Model file for the job. Use its own axes, mm. A direction names the side the tool comes from. Give positions to 0.01 mm unless a question says otherwise; leave off trailing zeros. Write each loop counter-clockwise with the first axis right and the second up, starting at its lowest first coordinate (ties: lowest second). Pieces come first, ordered by that corner, then holes.
```python
from build123d import *

# Parameters (mm, degrees)
SKETCH1_W           = 3.5
SKETCH1_H           = 1
SKETCH1_W_2         = 4
BOSS_EXTRUDE1_DEPTH = 1.3
SKETCH1_7_W         = 3.5
SKETCH1_7_H         = 1
BOSS_EXTRUDE3_DEPTH = 1
SKETCH1_8_W         = 4
SKETCH1_8_H         = 1
BOSS_EXTRUDE4_DEPTH = 1
FILLET2_R           = 1
SKETCH5_W           = 1.00602476
SKETCH5_H           = 0.93
BOSS_EXTRUDE5_DEPTH = 4
SKETCH7_W           = 1.00602476
SKETCH7_H           = 0.93
BOSS_EXTRUDE6_DEPTH = 3.5
BOSS_EXTRUDE7_DEPTH = 1
BOSS_EXTRUDE8_START = 1.3
BOSS_EXTRUDE8_DEPTH = 0.7
FILLET6_START       = -4.975
FILLET6_DEPTH       = 9.95
FILLET7_R           = 0.15
SKETCH10_W          = 0.9
SKETCH10_H          = 0.9
BOSS_EXTRUDE9_DEPTH = 4
CHAMFER2_SIZE       = 0.8
CHAMFER2_SIZE2      = 0.373046127
FILLET9_R           = 0.15
FILLET10_R          = 0.1
CHAMFER5_SIZE       = 1


with BuildPart() as part:
    # Sketch1 → Boss-Extrude1 (new body)
    # profile 1 of 4: a face of its own
    with BuildSketch(Plane(origin=(0, 0, 0), x_dir=(1, 0, 0), z_dir=(0, 1, 0))):
        with BuildLine():
            Line((0, 9.25), (-4.925, 9.25))
            Line((-4.925, 9.25), (-4.925, 8.25))
            Line((-4.925, 8.25), (-8.425, 8.25))
            Line((-8.425, 8.25), (-8.425, 9.25))
            Line((-8.425, 9.25), (-15.925, 9.25))
            ThreePointArc((-15.925, 9.25), (-18.399873734, 8.224873734), (-19.425, 5.75))
            Line((-19.425, 5.75), (-19.425, -8.25))
            ThreePointArc((-19.425, -8.25), (-19.132106781, -8.957106781), (-18.425, -9.25))
            Line((-18.425, -9.25), (-8, -9.25))
            Line((-8, -9.25), (-4.975, -9.25))
            Line((-4.975, -9.25), (-4.975, -9.15))
            Line((-4.975, -9.15), (-2, -9.15))
            Line((-2, -9.15), (-2, -8.75))
            Line((-2, -8.75), (-2, -8.25))
            Line((-2, -8.25), (-7.5, -8.25))
            ThreePointArc((-7.5, -8.25), (-8, -7.75), (-7.5, -7.25))
            Line((-7.5, -7.25), (7.5, -7.25))
            ThreePointArc((7.5, -7.25), (8, -7.75), (7.5, -8.25))
            Line((7.5, -8.25), (2, -8.25))
            Line((2, -8.25), (2, -8.75))
            Line((2, -8.75), (2, -9.15))
            Line((2, -9.15), (4.975, -9.15))
            Line((4.975, -9.15), (4.975, -9.25))
            Line((4.975, -9.25), (8, -9.25))
            Line((8, -9.25), (18.425, -9.25))
            ThreePointArc((18.425, -9.25), (19.132106781, -8.957106781), (19.425, -8.25))
            Line((19.425, -8.25), (19.425, 5.75))
            ThreePointArc((19.425, 5.75), (18.399873734, 8.224873734), (15.925, 9.25))
            Line((15.925, 9.25), (9.675, 9.25))
            Line((9.675, 9.25), (9.675, 8.25))
            Line((9.675, 8.25), (5.675, 8.25))
            Line((5.675, 8.25), (5.675, 9.25))
            Line((5.675, 9.25), (0, 9.25))
        make_face()
        with BuildLine():
            Line((-13.05, -6.65), (-14.5, -6.65))
            ThreePointArc((-14.5, -6.65), (-16.214733944, -5.939733944), (-16.925, -4.225))
            ThreePointArc((-16.925, -4.225), (-16.214733944, -2.510266056), (-14.5, -1.8))
            Line((-14.5, -1.8), (-13.05, -1.8))
            ThreePointArc((-13.05, -1.8), (-11.335266056, -2.510266056), (-10.625, -4.225))
            ThreePointArc((-10.625, -4.225), (-11.335266056, -5.939733944), (-13.05, -6.65))
        make_face(mode=Mode.SUBTRACT)
        with BuildLine():
            ThreePointArc((-16.925, 4.225), (-16.214733944, 5.939733944), (-14.5, 6.65))
            Line((-14.5, 6.65), (-13.05, 6.65))
            ThreePointArc((-13.05, 6.65), (-11.335266056, 5.939733944), (-10.625, 4.225))
            ThreePointArc((-10.625, 4.225), (-11.335266056, 2.510266056), (-13.05, 1.8))
            Line((-13.05, 1.8), (-14.5, 1.8))
            ThreePointArc((-14.5, 1.8), (-16.214733944, 2.510266056), (-16.925, 4.225))
        make_face(mode=Mode.SUBTRACT)
    # profile 2 of 4: a face of its own
    with BuildSketch(Plane(origin=(0, 0, 0), x_dir=(1, 0, 0), z_dir=(0, 1, 0))):
        with Locations((-6.675, 8.75)):
            Rectangle(SKETCH1_W, SKETCH1_H)
    # profile 3 of 4: a face of its own
    with BuildSketch(Plane(origin=(0, 0, 0), x_dir=(1, 0, 0), z_dir=(0, 1, 0))):
        with Locations((7.675, 8.75)):
            Rectangle(SKETCH1_W_2, SKETCH1_H)
    # profile 4 of 4: a face of its own
    with BuildSketch(Plane(origin=(0, 0, 0), x_dir=(1, 0, 0), z_dir=(0, 1, 0))):
        Polygon((-2, -8.75), (-2, -9.15), (2, -9.15), (2, -8.75), (2, -8.25), (-2, -8.25), align=None)
    extrude(amount=BOSS_EXTRUDE1_DEPTH)

    # Sketch1<7> → Boss-Extrude3 (add)
    with BuildSketch(Plane(origin=(0, 0, 0), x_dir=(1, 0, 0), z_dir=(0, 1, 0))):
        with Locations((-6.675, 8.75)):
            Rectangle(SKETCH1_7_W, SKETCH1_7_H)
    extrude(amount=-BOSS_EXTRUDE3_DEPTH)

    # Sketch1<8> → Boss-Extrude4 (add)
    with BuildSketch(Plane(origin=(0, 0, 0), x_dir=(1, 0, 0), z_dir=(0, 1, 0))):
        with Locations((7.675, 8.75)):
            Rectangle(SKETCH1_8_W, SKETCH1_8_H)
    extrude(amount=-BOSS_EXTRUDE4_DEPTH)

    # Fillet2
    fillet2_edges = [part.edges().sort_by_distance(p)[0] for p in [
        (7.675, -1, -8.25),
        (-6.675, -1, -8.25),
    ]]
    fillet(fillet2_edges, radius=FILLET2_R - 0.0001)  # a hair under: the kernel refuses the full size

    # Sketch5 → Boss-Extrude5 (add)
    with BuildSketch(Plane.ZY.offset(-9.675)):
        with Locations((-9.75301238, -0.535)):
            Rectangle(SKETCH5_W, SKETCH5_H)
    extrude(amount=BOSS_EXTRUDE5_DEPTH)

    # Sketch7 → Boss-Extrude6 (add)
    with BuildSketch(Plane.ZY.offset(8.425)):
        with Locations((-9.75301238, -0.535)):
            Rectangle(SKETCH7_W, SKETCH7_H)
    extrude(amount=-BOSS_EXTRUDE6_DEPTH)

    # Sketch1<12> → Boss-Extrude7 (add)
    with BuildSketch(Plane(origin=(0, 0, 0), x_dir=(1, 0, 0), z_dir=(0, 1, 0))):
        Polygon((-2, -8.75), (-2, -9.15), (2, -9.15), (2, -8.75), (2, -8.25), (-2, -8.25), align=None)
    extrude(amount=-BOSS_EXTRUDE7_DEPTH)

    # Sketch1<13> → Boss-Extrude8 (add)
    with BuildSketch(Plane(origin=(0, 0, 0), x_dir=(1, 0, 0), z_dir=(0, 1, 0)).offset(BOSS_EXTRUDE8_START)):
        Polygon((-4.975, -9.15), (-4.975, -9.25), (0, -9.25), (4.975, -9.25), (4.975, -9.15), (2, -9.15), (-2, -9.15), align=None)
    extrude(amount=-BOSS_EXTRUDE8_DEPTH)

    # Fillet6: read off the stored shape, not the designer's step
    # Fillet6 outline → Fillet6 (add)
    with BuildSketch(Plane.YZ.offset(FILLET6_START)):
        with BuildLine():
            Line((0.6, 9.15), (0.6, 9.25))
            add(Edge.make_bspline(
                [(0.6, 9.25), (0.59163758, 9.15), (0.002086963, 9.15)],
                knots=[0, 0, 0, 1, 1, 1], degree=2, weights=[1, 0.735980072, 1]))
            Line((0.002086963, 9.15), (0.6, 9.15))
        make_face()
    extrude(amount=FILLET6_DEPTH)

    # Fillet7
    # the kernel refuses this fillet: 0.15 mm, written as the material it adds along each edge
    with BuildSketch(Plane(origin=(-4.975, 0, 9.15), x_dir=(1, 0, 0), z_dir=(0, 1, 0))) as fillet7_piece_1:
        with BuildLine():
            CenterArc((0.141421356, -0.15), FILLET7_R, 90, 70.528779366)
            Line((0, -0.1), (-0.002828427, -0.099))
            ThreePointArc((-0.002828427, -0.099), (-0.003, -0.05), (-0.003, 0))
            Line((-0.003, 0), (0, 0.003))
            Line((0, 0.003), (0.141421356, 0.003))
            Line((0.141421356, 0.003), (0.141421356, 0))
        make_face()
    extrude(amount=0.603127727)
    with BuildSketch(Plane(origin=(4.975, 0, 9.15), x_dir=(0, 0, 1), z_dir=(0, 1, 0))) as fillet7_piece_2:
        with BuildLine():
            CenterArc((0.15, -0.141421356), FILLET7_R, 109.471220634, 70.528779366)
            Line((0, -0.141421356), (-0.003, -0.141421356))
            Line((-0.003, -0.141421356), (-0.003, 0))
            Line((-0.003, 0), (0, 0.003))
            ThreePointArc((0, 0.003), (0.05, 0.003), (0.099, 0.002828427))
            Line((0.099, 0.002828427), (0.1, 0))
        make_face()
    extrude(amount=0.603127727)

    # Sketch10 → Boss-Extrude9 (add)
    with BuildSketch(Plane(origin=(2, 0, 0), x_dir=(0, 0, -1), z_dir=(1, 0, 0))):
        with Locations((-9.6, -0.55)):
            Rectangle(SKETCH10_W, SKETCH10_H)
    extrude(amount=-BOSS_EXTRUDE9_DEPTH)

    # Chamfer2
    chamfer2_edges = [part.edges().sort_by_distance(p)[0] for p in [
        (0, -1, 10.05),
    ]]
    chamfer2_side = [part.faces().sort_by_distance(p)[0] for p in [
        (0, -1, 9.15),
    ]]
    chamfer(chamfer2_edges, length=CHAMFER2_SIZE, length2=CHAMFER2_SIZE2, reference=chamfer2_side[0])

    # Fillet9
    fillet9_edges = [part.edges().sort_by_distance(p)[0] for p in [
        (-2, -0.5, 8.25),
        (2, -0.5, 8.25),
        (0, -1, 8.25),
        (2, -1, 8.75),
        (-2, -1, 8.75),
    ]]
    fillet(fillet9_edges, radius=FILLET9_R)

    # Fillet10
    fillet10_edges = [part.edges().sort_by_distance(p)[0] for p in [
        (0, -0.1, 10.05),
        (0, -0.626953873, 10.05),
    ]]
    fillet(fillet10_edges, radius=FILLET10_R)

    # Chamfer5
    chamfer5_edges = [part.edges().sort_by_distance(p)[0] for p in [
        (-10.625, 1.3, -4.225),
        (-13.775, 1.3, -1.8),
        (-16.925, 1.3, -4.225),
        (-13.775, 1.3, -6.65),
        (-16.925, 1.3, 4.225),
        (-13.775, 1.3, 1.8),
        (-10.625, 1.3, 4.225),
        (-13.775, 1.3, 6.65),
    ]]
    chamfer(chamfer5_edges, length=CHAMFER5_SIZE)


solid = part.part
```
1. Slice it at A-A, the plane x = 12. Write the cut outline in (y, z).
Calculated:
outline: (0, -9.25) - (1.3, -9.25) - (1.3, 9.25) - (0, 9.25) - close
2. Probe probe 1 along Z at (x, y) = (-6, 0.1); probe 2 along Y at (x, z) = (1, 3.5); probe 3 along Z at (x, y) = (2, 0.2). List the from-to ranges inside material, lowest first.
Calculated:
probe 1: z = -9.25 to 7.25, 8.25 to 9.25
probe 2: y = 0 to 1.3
probe 3: z = -9.25 to 7.25, 8.25 to 9.16
3. Which spindle directions (+Z, -Z, +X, -X, +Y, -Y) get a long thin tool onto all of the face, cutting with end or side? Do faces 1 (the cylindrical face through (-8, 0.64, 7.76)), 2 (the flat face through (-13.76, 0.81, 7.16)), 3 (the flat face through (-4.925, -0.5, -9.3)), 4 (the flat face through (9.675, -0.5, -9.3)). Say none if no direction does.
Calculated:
face 1: +Y, -Y
face 2: +Y
face 3: +Z, -Z, -Y
face 4: +Z, -Z, +X, -Y
4. Pull direction X, two halves, no side cores. Call faces 5 (the cylindrical face through (-18.373, 0.641, -8.252)), 6 (the flat face through (0, 1, -9.25)), 7 (the flat face through (0, 1, 7.25)), 8 (the cylindrical face through (18.427, 0.641, -8.198)): +X half, -X half, draft (parallel to the pull), parting line (faces both ways), or undercut.
Calculated:
face 5: -X half
face 6: draft
face 7: undercut
face 8: +X half
5. Pin check, flat tips, straight feed: P1, Ø1, axis at x = -1.5, y = 0, coming from the -Z side; P2, Ø1, axis at x = -2.5, y = 0.5, coming from the +Z side; P3, Ø0.5, axis at x = -6, z = -10, coming from the +Y side. Stop position of each tip, or through.
Calculated:
P1: stops at z = -9.25
P2: stops at z = 9.25
P3: stops at y = -0.07
